Check sheet for the modelled part. Datum: model origin and axes. Units: mm. A direction names the side the tool comes from. Coordinates: 2 decimals unless noted, no trailing zeros. Use CSV: the item, a comma, the result in double quotes. Start each with the question number.
1. Gauge pin test, flat ends, axial feed: pin 1 (1.2 mm diameter, centred on y = -2.5, z = 0.5, fed in from +X); pin 2 (2 mm diameter, centred on x = 14, z = -9, fed in from -Y); pin 3 (5 mm diameter, centred on y = -1.5, z = 7, fed in from +X); pin 4 (5 mm diameter, centred on x = -5.66, z = 5.66, fed in from +Y). Record the tip position at first contact, or that the pin passes through.
2. Thickness scan on L1, parallel to Z at x = 0, y = 3; L2, parallel to Z at x = 0, y = 8.5; L3, parallel to X at y = 0.5, z = -6.5. Record the ranges inside material, lowest first.
3. Release check for a two-part mould opening along Z. For faces 1 (the face through (-14, -2, -2)), 2 (the face through (0, -2, 15.2)), 3 (the face through (-0.3, 12.5, -4.3)), 4 (the face through (0, 6, -6)) record: pulls with the +Z half, pulls with the -Z half, needs draft (parallel to the pull), parting line crosses it, or undercut.
4. Set-up check for faces 5 (the face through (0, -2, -13.2)), 6 (the face through (2, -2, 14)), 7 (the face through (14, -2, 2)), 8 (the face through (-13.2, -2, 0)), 9 (the face through (-22, 7.5, -2)): record each of +Z, -Z, +X, -X, +Y, -Y from which the full face is reachable in a straight line by a thin tool's end or side.
5. Sectioned sample at A-A, the plane x = 0. Count the separate pieces of the cut face and the enclosed holes in it, and give its area (4 significant figures).
Autodesk Inventor part; units mm, degrees
ref_plane "YZ Plane" through (0, 0, 0) normal (1, 0, 0) x (0, 1, 0)
ref_plane "XZ Plane" through (0, 0, 0) normal (0, 1, 0) x (-1, 0, 0)
ref_plane "XY Plane" through (0, 0, 0) normal (0, 0, 1) x (1, 0, 0)
sketch "Эскиз1" plane through (0, 0, 0) normal (0, 1, 0) x (-1, 0, 0)
  circle A0 centre (0, 0) radius 17.5
  dimension "d0" = 35
extrude "Выдавливание1" add sketch "Эскиз1" along normal blind 7.5
sketch "Эскиз2" plane through (0, 7.5, 0) normal (0, 1, 0) x (1, 0, 0)
  circle A0 centre (0, 0) radius 22.5
  dimension "d3" = 45
extrude "Выдавливание2" add sketch "Эскиз2" along normal blind 5
fillet "Сопряжение1" radius 4.25 1 edges at (17.5, 7.5, 0)
fillet "Сопряжение2" radius 4.25 1 edges at (-22.5, 12.5, 0)
sketch "Эскиз3" plane through (0, 0, 0) normal (0, -1, 0) x (1, 0, 0)
  line L0 (-24.85, 5.95) -> (-15.15, 5.95)
  line L1 (-15.15, 5.95) -> (-15.15, -5.95)
  line L2 (-15.15, -5.95) -> (-24.85, -5.95)
  line L3 (-24.85, -5.95) -> (-24.85, 5.95)
  line L4 (-4.7, 15.3) -> (-4.7, 25)
  line L5 (-4.7, 25) -> (5, 25)
  line L6 (5, 25) -> (5, 15.3)
  line L7 (5, 15.3) -> (-4.7, 15.3)
  line L8 (5, -15.3) -> (5, -25)
  line L9 (5, -25) -> (-4.7, -25)
  line L10 (-4.7, -25) -> (-4.7, -15.3)
  line L11 (-4.7, -15.3) -> (5, -15.3)
  line L12 (15.15, 5.95) -> (24.85, 5.95)
  line L13 (24.85, 5.95) -> (24.85, -5.95)
  line L14 (24.85, -5.95) -> (15.15, -5.95)
  line L15 (15.15, -5.95) -> (15.15, 5.95)
  circle A0 centre (0, 8) radius 2
  circle A1 centre (-5.6569, -5.6569) radius 2
  circle A2 centre (0, -8) radius 2
  circle A3 centre (0, 0) radius 4
  circle A4 centre (8, 0) radius 2
  circle A5 centre (-8, 0) radius 2
  circle A6 centre (5.6569, -5.6569) radius 2
  circle A7 centre (-5.6569, 5.6569) radius 2
  circle A8 centre (5.6569, 5.6569) radius 2
  circle A9 centre (0, 0) radius 35
extrude "Выдавливание3" cut sketch "Эскиз3" against normal through all contours A0 | A1 | A2 | A3 | A4 | A5 | A6 | A7 | A8
sketch "Эскиз4" plane through (0, 0, 0) normal (0, -1, 0) x (1, 0, 0)
  circle A0 centre (-8, 0) radius 2
  line L0 (-8, 0) -> (-13.2, 0)
  line L1 (-13.2, 0) -> (-13.2, -2)
  line L2 (-13.2, -2) -> (-15.2, -2)
  line L3 (-15.2, -2) -> (-15.2, 2)
  line L4 (-15.2, 2) -> (-13.2, 2)
  line L5 (-13.2, 2) -> (-13.2, 0)
  line L6 (2, -15.2) -> (-2, -15.2)
  line L7 (2, -13.2) -> (2, -15.2)
  line L8 (-2, -13.2) -> (0, -13.2)
  line L9 (0, -13.2) -> (2, -13.2)
  line L10 (-2, -15.2) -> (-2, -13.2)
  line L11 (15.2, 2) -> (15.2, -2)
  line L12 (13.2, 2) -> (15.2, 2)
  line L13 (13.2, -2) -> (13.2, 0)
  line L14 (13.2, 0) -> (13.2, 2)
  line L15 (15.2, -2) -> (13.2, -2)
  line L16 (-2, 15.2) -> (2, 15.2)
  line L17 (-2, 13.2) -> (-2, 15.2)
  line L18 (2, 13.2) -> (0, 13.2)
  line L19 (0, 13.2) -> (-2, 13.2)
  line L20 (2, 15.2) -> (2, 13.2)
  point P0 (0, 0)
  dimension "d10" = 5.2
  dimension "d11" = 2
  dimension "d12" = 4
  dimension "d15" = 360
extrude "Выдавливание4" add sketch "Эскиз4" along normal blind 4.5 contours L1 L2 L3 L4 L5 | L6 L10 L8 L9 L7 | L11 L15 L13 L14 L12 | L16 L20 L18 L19 L17
sketch "Эскиз6" plane through (0, 0, 0) normal (0, -1, 0) x (1, 0, 0)
  circle A0 centre (0, 0) radius 17.5
  point P0 (0, 17.5)
ref_plane "РабПлоскость1" through (0, 0, 17.5) normal (0, 0, 1) x (1, 0, 0)
sketch "Эскиз7" plane through (0, 0, 17.5) normal (0, 0, 1) x (1, 0, 0)
  line L0 (17.5, 3.25) -> (-17.5, 3.25)
  circle A0 centre (-12.5, 3.25) radius 2.2
  line L1 (-17.5, 0) -> (-17.5, 3.25)
  dimension "d22" = 4.4
  dimension "d23" = 5
extrude "Выдавливание5" cut sketch "Эскиз7" against normal through all
properties part number "мини катушка3"
Completed:
1,pin 1,"x = 15.2"
1,pin 2,"y = 0"
1,pin 3,"x = 16.77"
1,pin 4,"y = 12.5"
2,L1,"-17.5 to -10, -6 to -4, 4 to 6, 10 to 17.5"
2,L2,"-22.49 to -10, -6 to -4, 4 to 6, 10 to 22.49"
2,L3,"-16.25 to -7.47, -3.84 to -1.32, 1.32 to 3.84, 7.47 to 16.25"
3,face 1,"pulls with the -Z half"
3,face 2,"pulls with the +Z half"
3,face 3,"needs draft"
3,face 4,"undercut"
4,face 5,"+X, -X, -Y"
4,face 6,"+Z, -Z, +X, -Y"
4,face 7,"+Z, +X, -X, -Y"
4,face 8,"+Z, -Z, -Y"
4,face 9,"-Y"
5,separate pieces,"4"
5,enclosed holes,"0"
5,area,"305.5 mm²"
